```python
from build123d import *

# Parameters (mm, degrees)
BOSS_EXTRUDE1_START     = -26
SKETCH1_R               = 1.25
BOSS_EXTRUDE1_DEPTH     = 29
SKETCH2_R               = 1.05
CUT_EXTRUDE1_DEPTH      = 65.100019501
FILLET1_R               = 2.2
CUT_EXTRUDE2_DEPTH      = 63.8694083
CUT_EXTRUDE2_DEPTH_BACK = 63.8694083
SKETCH3_W               = 60
SKETCH3_H               = 23.2
CUT_EXTRUDE3_DEPTH      = 63.8694083
CUT_EXTRUDE3_DEPTH_BACK = 63.8694083
SKETCH4_W               = 23.2
SKETCH4_H               = 30.3
FILLET2_R               = 2.2


with BuildPart() as part:
    # Sketch1 → Boss-Extrude1 (new body)
    with BuildSketch(Plane.XY.offset(BOSS_EXTRUDE1_START)):
        Polygon((-30, -30), (-30, 2.5), (-22, 2.5), (-22, -2.5), (-17, -2.5), (-17, 2.5), (0, 2.5), (0, 7.5), (-35, 7.5), (-35, -25), (-48.75, -25), (-48.75, -30), align=None)
        with Locations((-19.5, 0)):
            Circle(SKETCH1_R, mode=Mode.SUBTRACT)
    boss_extrude1 = extrude(amount=BOSS_EXTRUDE1_DEPTH)

    # Sketch2 → Cut-Extrude1 (cut, through all)
    with BuildSketch(Plane(origin=(0, -25, 0), x_dir=(1, 0, 0), z_dir=(0, 1, 0))):
        with Locations(Location((-45, 23, 0), (0, 0, 180))):
            Circle(SKETCH2_R)
        with Locations(Location((-45, 0, 0), (0, 0, 180))):
            Circle(SKETCH2_R)
    cut_extrude1 = extrude(amount=-CUT_EXTRUDE1_DEPTH, mode=Mode.SUBTRACT)

    # Mirror1: Boss-Extrude1, Cut-Extrude1 across plane
    add(boss_extrude1.mirror(Plane(origin=(0, 0, 0), x_dir=(0, 0, 1), z_dir=(1, 0, 0))))
    add(cut_extrude1.mirror(Plane(origin=(0, 0, 0), x_dir=(0, 0, 1), z_dir=(1, 0, 0))), mode=Mode.SUBTRACT)

    # Fillet1
    fillet1_edges = [part.edges().sort_by_distance(p)[0] for p in [
        (-17, -2.5, -11.5),
        (-22, -2.5, -11.5),
        (-22, 2.5, -11.5),
        (-30, 2.5, -11.5),
        (-30, -30, -11.5),
        (-35, -25, -11.5),
        (-35, 7.5, -11.5),
        (-48.75, -27.5, 3),
        (-48.75, -27.5, -26),
        (17, -2.5, -11.5),
        (22, -2.5, -11.5),
        (22, 2.5, -11.5),
        (30, 2.5, -11.5),
        (30, -30, -11.5),
        (48.75, -27.5, -26),
        (48.75, -27.5, 3),
        (35, -25, -11.5),
        (35, 7.5, -11.5),
    ]]
    fillet(fillet1_edges, radius=FILLET1_R)

    # Sketch3 → Cut-Extrude2 (cut, two sides: drawn at the far end of the back side and taken through both)
    with BuildSketch(Plane(origin=(0, 0, 0), x_dir=(1, 0, 0), z_dir=(0, 1, 0)).offset(-CUT_EXTRUDE2_DEPTH_BACK)):
        with Locations((0, 11.5)):
            Rectangle(SKETCH3_W, SKETCH3_H)
    extrude(amount=CUT_EXTRUDE2_DEPTH + CUT_EXTRUDE2_DEPTH_BACK, mode=Mode.SUBTRACT)

    # Sketch4 → Cut-Extrude3 (cut, two sides: drawn at the far end of the back side and taken through both)
    with BuildSketch(Plane(origin=(0, 0, 0), x_dir=(0, 0, -1), z_dir=(1, 0, 0)).offset(-CUT_EXTRUDE3_DEPTH_BACK)):
        with Locations((11.5, -9.85)):
            Rectangle(SKETCH4_W, SKETCH4_H)
    extrude(amount=CUT_EXTRUDE3_DEPTH + CUT_EXTRUDE3_DEPTH_BACK, mode=Mode.SUBTRACT)

    # Fillet2
    fillet2_edges = [part.edges().sort_by_distance(p)[0] for p in [
        (-30, -25, -11.5),
        (30, -25, -11.5),
    ]]
    fillet(fillet2_edges, radius=FILLET2_R)


solid = part.part
```
Check sheet for the modelled part. Datum: model origin and axes. Units: mm. A direction names the side the tool comes from. Round coordinates to 2 decimals unless told otherwise and drop trailing zeros. Order: outer loops, then holes, each group sorted by start corner. A loop starts at its lowest first (then second) coordinate and runs counter-clockwise, first axis right, second up. Notation, with made-up numbers: (73, 23) - (100, 23) arc R20 ccw to (100, 39) - close; hole circle Ø2 at (-38.75, 17). An arc over 180 degrees is marked (long way). Answer as CSV lines item,"result". Start each with the question number.
1) Tool access check on faces 1 (the face through (22.66, 1.87, -24.53)), 2 (the face through (-30.63, -25.66, -11.66)), 3 (the face through (-30, 6, -12)). Record the directions out of +Z, -Z, +X, -X, +Y, -Y that give a thin tool (end or side, any length) a straight path to the whole face; none if there is none.
2) Scan lines: probe 1 along Z at (x, y) = (-45, -28); probe 2 along X at (y, z) = (-27.95, -23); probe 3 along Y at (x, z) = (-19.5, 1.45). Record each from-to range of solid material in increasing order.
3) Depth check by flat-ended pin: pin 1 (0.5 mm diameter, centred on y = 0, z = 1, fed in from +X); pin 2 (0.5 mm diameter, centred on x = -19.5, z = -24, fed in from -Y); pin 3 (1.4 mm diameter, centred on y = 0.5, z = -24.5, fed in from -X); pin 4 (2.5 mm diameter, centred on x = -45, z = 0, fed in from -Y). Enter the tip coordinate at first touch or a pass-through.
4) Draft check along Z on faces 4 (the face through (0, 3, 0.1)), 5 (the face through (21.37, -1.84, -24.53)), 6 (the face through (-3, 3, 3)). Enter one of: +Z half, -Z half, draft (parallel to the pull), parting line (faces both ways), or undercut.
5) Section check A-A (y = -9). Record the cut outline in (x, z), then the cut area to 3 significant figures.
6) Section check D-D (x = -29). Record the cut outline in (y, z), then the cut area to 3 significant figures.
7) Section check B-B (x = -45). Record the cut outline in (y, z), then the cut area to 3 significant figures.
8) Section check C-C (z = -4.75). Record the cut outline in (x, y).
Determined:
1,face 1,"+Z, -Z, -Y"
1,face 2,"none"
1,face 3,"+Y, -Y"
2,probe 1,"-26 to -24.05, -21.95 to -1.05, 1.05 to 3"
2,probe 2,"-48.75 to -46.05, -43.95 to -30.01, 30.01 to 43.95, 46.05 to 48.75"
2,probe 3,"-2.5 to -1.25, 1.25 to 7.5"
3,pin 1,"x = 35"
3,pin 2,"y = -2.5"
3,pin 3,"x = -35"
3,pin 4,"y = -30"
4,face 4,"undercut"
4,face 5,"draft"
4,face 6,"+Z half"
5,outline,"(-35, -26) - (-30, -26) - (-30, -23.1) - (-35, -23.1) - close; (-35, 0.1) - (-30, 0.1) - (-30, 3) - (-35, 3) - close; (30, -26) - (35, -26) - (35, -23.1) - (30, -23.1) - close; (30, 0.1) - (35, 0.1) - (35, 3) - (30, 3) - close"
5,area,"58.0 mm^2"
6,outline,"(2.14, -26) - (7.5, -26) - (7.5, -23.1) - (2.14, -23.1) - close; (2.14, 0.1) - (7.5, 0.1) - (7.5, 3) - (2.14, 3) - close"
6,area,"31.1 mm^2"
7,outline,"(-30, -26) - (-25, -26) - (-25, -24.05) - (-30, -24.05) - close; (-30, -21.95) - (-25, -21.95) - (-25, -1.05) - (-30, -1.05) - close; (-30, 1.05) - (-25, 1.05) - (-25, 3) - (-30, 3) - close"
7,area,"124 mm^2"
8,outline,"(-48.75, -30) - (-32.2, -30) arc R2.2 ccw to (-30, -27.8) - (-30, -27.2) arc R2.2 ccw to (-32.2, -25) - (-48.75, -25) - close; (-35, 5.3) - (-30, 5.3) - (-30, 7.5) - (-32.8, 7.5) arc R2.2 ccw to start; (30, -27.8) arc R2.2 ccw to (32.2, -30) - (48.75, -30) - (48.75, -25) - (32.2, -25) arc R2.2 ccw to (30, -27.2) - close; (30, 5.3) - (35, 5.3) arc R2.2 ccw to (32.8, 7.5) - (30, 7.5) - close"
